Read the model definition and answer for the solid it produces. Units are mm, in the model's axes. Face numbers are marked on the shaded views. A direction names the side the tool comes from. Coordinates: 2 decimals unless noted, no trailing zeros. Loops run counter-clockwise (first coordinate to the right, second up) from the corner with the lowest first, then second, coordinate; pieces in that order, holes last.
from build123d import *

# Parameters (mm, degrees)
BASE_FLANGE1_DEPTH = 20
SKETCH6_R          = 3
CUT_EXTRUDE1_DEPTH = 44.874821937
FILLET1_R          = 10
FILLET2_R          = 5
SKETCH7_R          = 3
CUT_EXTRUDE2_DEPTH = 42.768177181


# Read off the part's stored shape, not the designer's step: Base-Flange1
with BuildPart() as part:
    # Base-Flange1 outline → Base-Flange1 (new body)
    with BuildSketch(Plane.XY):
        with BuildLine():
            Line((4.175, 26.825), (25, 26.825))
            Line((25, 26.825), (25, 30))
            Line((25, 30), (4.175, 30))
            ThreePointArc((4.175, 30), (1.222829189, 28.777170811), (0, 25.825))
            Line((0, 25.825), (0, 0))
            Line((0, 0), (3.175, 0))
            Line((3.175, 0), (3.175, 25.825))
            ThreePointArc((3.175, 25.825), (3.467893219, 26.532106781), (4.175, 26.825))
        make_face()
    extrude(amount=BASE_FLANGE1_DEPTH)

    # Sketch6 → Cut-Extrude1 (cut, through all)
    with BuildSketch(Plane.ZY):
        with Locations((10, 10)):
            Circle(SKETCH6_R)
    extrude(amount=-CUT_EXTRUDE1_DEPTH, mode=Mode.SUBTRACT)

    # Fillet1
    fillet1_edges = [part.edges().sort_by_distance(p)[0] for p in [
        (1.5875, 0, 0),
        (1.5875, 0, 20),
    ]]
    fillet(fillet1_edges, radius=FILLET1_R - 0.0001)  # a hair under: the kernel refuses the full size

    # Fillet2
    fillet2_edges = [part.edges().sort_by_distance(p)[0] for p in [
        (25, 28.4125, 20),
        (25, 28.4125, 0),
    ]]
    fillet(fillet2_edges, radius=FILLET2_R)

    # Sketch7 → Cut-Extrude2 (cut, through all)
    with BuildSketch(Plane.XZ.offset(-26.825)):
        with Locations(Location((9.175, 7, 0), (0, 0, 270))):
            Circle(SKETCH7_R)
        with Locations(Location((19, 13, 0), (0, 0, 270))):
            Circle(SKETCH7_R)
    extrude(amount=-CUT_EXTRUDE2_DEPTH, mode=Mode.SUBTRACT)


solid = part.part
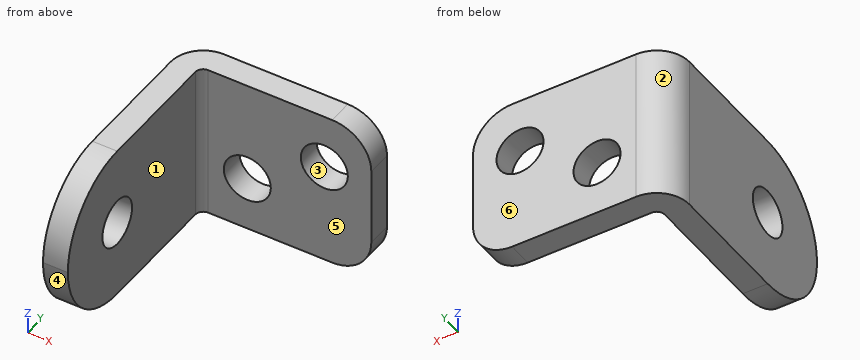
Q1. Determine the mould class of the marked faces 1, 2, 3 and 4 for opening direction X: +X half, -X half, draft (parallel to the pull), parting line (faces both ways), or undercut.
Findings below:
face 1: +X half
face 2: -X half
face 3: undercut
face 4: draft
Q2. A cutting plane is placed at A-A (y = 7.75). Give the vertices of the cut face in (x, z) (3 decimals), then the cut area to 3 significant figures.
Findings below:
outline: (0, 0.256) - (3.175, 0.256) - (3.175, 8.016) - (0, 8.016) - close; (0, 11.984) - (3.175, 11.984) - (3.175, 19.744) - (0, 19.744) - close
area: 49.3 mm2
Q3. A cutting plane is placed at C-C (z = 11.25). Give the vertices of the cut face in (x, y) (3 decimals), then the cut area to 3 significant figures.
Findings below:
outline: (0, 0.078) - (3.175, 0.078) - (3.175, 7.273) - (0, 7.273) - close; (0, 12.727) - (3.175, 12.727) - (3.175, 25.825) arc R1 cw to (4.175, 26.825) - (16.563, 26.825) - (16.563, 30) - (4.175, 30) arc R4.175 ccw to (0, 25.825) - close; (21.437, 26.825) - (25, 26.825) - (25, 30) - (21.437, 30) - close
area: 128 mm2
Q4. A cutting plane is placed at B-B (x = 20.75). Give the vertices of the cut face in (y, z) (3 decimals), then the cut area to 3 significant figures.
Findings below:
outline: (26.825, 0.057) - (30, 0.057) - (30, 10.563) - (26.825, 10.563) - close; (26.825, 15.437) - (30, 15.437) - (30, 19.943) - (26.825, 19.943) - close
area: 47.7 mm2
Q5. Flat-ended cylindrical pins translate along their axes: pin 1 Ø6 at (x, z) = (9.5, 10) entering from -Y (3 decimals); pin 2 Ø10 at (y, z) = (20, 17) entering from +X (3 decimals); pin 3 Ø6 at (x, z) = (11, 7) entering from +Y. Find the tip coordinate at first contact, or state that the pin passes through.
Findings below:
pin 1: stops at y = 26.825
pin 2: stops at x = 3.175
pin 3: stops at y = 30
Q6. A cutting plane is placed at D-D (z = 13.5). Give the vertices of the cut face in (x, y) (3 decimals).
Findings below:
outline: (0, 0.632) - (3.175, 0.632) - (3.175, 25.825) arc R1 cw to (4.175, 26.825) - (16.042, 26.825) - (16.042, 30) - (4.175, 30) arc R4.175 ccw to (0, 25.825) - close; (21.958, 26.825) - (25, 26.825) - (25, 30) - (21.958, 30) - close
Q7. Straight lines are drawn through the part: probe 1 along Y at (x, z) = (21.5, 17.5) (3 decimals); probe 2 along X at (y, z) = (12, 1.25) (3 decimals); probe 3 along Z at (x, y) = (9.75, 28.75). For each, find the intervals that lie inside material, in ascending order.
Findings below:
probe 1: y = 26.825 to 30
probe 2: x = 0 to 3.175
probe 3: z = 0 to 4.06, 9.94 to 20
Q8. Which of the six approach directions +Z, -Z, +X, -X, +Y, -Y give full straight-line access (tool end or side, diameter ignored) to the marked faces 5 and 6?
Findings below:
face 5: +Z, -Z, +X, -Y
face 6: +Z, -Z, +X, -X, +Y
